Autodesk Inventor part; units mm, degrees
ref_plane "YZ Plane" through (0, 0, 0) normal (1, 0, 0) x (0, 1, 0)
ref_plane "XZ Plane" through (0, 0, 0) normal (0, 1, 0) x (-1, 0, 0)
ref_plane "XY Plane" through (0, 0, 0) normal (0, 0, 1) x (1, 0, 0)
sketch "Sketch1" plane through (0, 0, 0) normal (0, 0, 1) x (1, 0, 0)
  circle A0 centre (0, 0) radius 11.4
  line L0 (-15, 17.5) -> (15, 17.5)
  line L1 (15, 17.5) -> (15, -17.5)
  line L2 (15, -17.5) -> (-15, -17.5)
  line L3 (-15, -17.5) -> (-15, 17.5)
  line L4 (-15, 17.5) -> (15, -17.5) construction
  line L5 (15, 17.5) -> (-15, -17.5) construction
  dimension "d0" = 22.8
  dimension "d1" = 30
  dimension "d2" = 35
extrude "Extrusion1" add sketch "Sketch1" along normal blind 25
sketch "Sketch3" plane through (-15, 17.5, 0) normal (0, 1, 0) x (1, 0, 0)
  line L0 (30, 0) -> (0, 0)
  line L1 (0, 0) -> (30, -25)
  line L2 (45, 40) -> (-15, 40)
  line L3 (-15, 40) -> (-15, -25)
  line L4 (-15, -25) -> (45, -25)
  line L5 (45, -25) -> (45, 40)
  line L6 (0, 0) -> (30, 0)
  line L7 (30, 0) -> (45, 0)
  line L8 (30, -25) -> (0, -25)
  point P0 (15, 0)
  point P1 (15, -12.5)
  dimension "d8" = 60
  dimension "d9" = 65
  dimension "d27" = 0
extrude "Extrusion3" add sketch "Sketch3" along normal blind 6
sketch "Sketch4" plane through (-15, 23.5, 0) normal (0, 1, 0) x (1, 0, 0)
  line L0 (-15, 33) -> (45, 33)
  line L1 (-15, 27) -> (45, 27)
  line L2 (45, 33) -> (45, 27)
  line L3 (-15, 27) -> (-15, 33)
  line L4 (45, 40) -> (-15, 40)
  dimension "d20" = 7
  dimension "d21" = 13
sketch "Sketch5" plane through (0, 0, 25) normal (0, 0, 1) x (1, 0, 0)
  circle A0 centre (0, 0) radius 11.4
  circle A1 centre (0, 0) radius 8.5
  dimension "d24" = 17
extrude "Extrusion5" add sketch "Sketch5" against normal blind 3
chamfer "Chamfer1" distance 5 angle 45 3 edges at (15, 17.5, 12.5) (-15, 17.5, 12.5) (0, 17.5, 0)
extrude "Extrusion6" add sketch "Sketch4" along normal blind 1.5
sketch "Sketch8" plane through (-15, 23.5, 0) normal (0, 1, 0) x (1, 0, 0)
  line L0 (45, 40) -> (-15, 40)
  line L1 (-15, 20) -> (45, 20)
  line L2 (45, 20) -> (45, 14)
  line L3 (45, 14) -> (-15, 14)
  line L4 (-15, 14) -> (-15, 20)
  point P0 (43, 40)
  point P1 (-13, 40)
  point P2 (15, 11.0426)
  dimension "d47" = 6
  dimension "d50" = 20
extrude "Extrusion7" add sketch "Sketch8" along normal blind 20
sketch "Sketch10" plane through (-15, 25, 0) normal (0, 1, 0) x (1, 0, 0)
  line L0 (45, 33) -> (-15, 33)
  line L1 (15, 33) -> (15, 27)
  line L2 (45, 27) -> (-15, 27)
  line L3 (0, 33) -> (0, 27)
  line L4 (30, 33) -> (30, 27)
  point P0 (15, 0)
  point P1 (0, 30)
  point P2 (30, 30)
  dimension "d51" = 15
  dimension "d52" = 15
hole "Hole2" at (-15, 25, -30) at (15, 25, -30) direction (0, -1, 0) diameter 5.5 end through all counterbore diameter 10 counterbore depth 1.5
sketch "Sketch11" plane through (30, 23.5, -20) normal (0, 0, -1) x (-1, 0, 0)
  line L0 (60, 0) -> (60, 20)
  line L1 (60, 10) -> (0, 10)
  line L2 (0, 0) -> (0, 20)
  line L3 (60, 20) -> (0, 20)
  line L4 (30, 20) -> (30, 10)
  point P0 (30, -23.5)
hole "Hole3" at (0, 33.5, -20) direction (0, 0, 1) diameter 5.5 end through all
fillet "Fillet2" radius 2 10 edges at (-30, 20.5, -40) (30, 20.5, -40) (-30, 20.5, 25) (30, 20.5, 25) (30, 43.5, -17) (-30, 43.5, -17) (-15, -17.5, 12.5) (15, -17.5, 12.5) (0, -17.5, 25) (0, -17.5, 0)
properties part number "Estrutura - Suporte Rolamento Z Motor"
Design review of the part built by this model. Coordinates are the model's own, in mm. A direction names the side the tool comes from. Round coordinates to 2 decimals unless told otherwise and drop trailing zeros. Order: outer loops, then holes, each group sorted by start corner. A loop starts at its lowest first (then second) coordinate and runs counter-clockwise, first axis right, second up. Notation, with made-up numbers: M 19,11 L 47,11 A12 cw 47,28 Z; hole C 76,8.25 d7. An arc over 180 degrees is marked long. Answer as CSV lines item,"result". Start each with the question number.
1) Wall thickness on line 1 along X through (y, z) = (18, -30); line 2 along Y through (x, z) = (0, -15); line 3 along Z through (x, y) = (15, 21.9): over which ranges is each line inside the solid? List them lowest first. Write a range as [from, to].
2) Add section D-D (z = -2). Give the boundary of the cut face in (x, y).
3) For pin 1 Ø19.5 at (x, y) = (0, 0) entering from -Z; pin 2 Ø20 at (y, z) = (5, 8.5) entering from +X; pin 3 Ø6 at (x, z) = (-21, -29) entering from -Y, all flat-tipped, find the tip position at first contact; note any pin that passes through.
4) The part is to be moulded in two halves that separate along X. For faces 4 (the face through (-25, 25, -30)), 5 (the face through (15, -1, 12)), 6 (the face through (-9, 7, 11)), say which applies: +X half, -X half, draft (parallel to the pull), parting line (faces both ways), or undercut.
5) Add section C-C (x = -6). Give the boundary of the cut face in (y, z).
6) Add section A-A (y = 0). Give the boundary of the cut face in (x, z), then the cut area to 3 significant figures.
7) Add section B-B (x = 0). Give the number of separate pieces and of enclosed holes in the cut face, then the cut area to 3 significant figures.
8) Tool access review of faces 1 (the face through (0, 25, -30)), 2 (the face through (-4, -8, 22)), 3 (the face through (-7, -11, 0)): name each direction out of +Z, -Z, +X, -X, +Y, -Y from which nothing blocks a thin tool from reaching the whole face with its end or side.
Resolved:
1,line 1,"[-30, -17.75], [-12.25, 12.25], [17.75, 30]"
1,line 2,"[17.5, 30.75], [36.25, 43.5]"
1,line 3,"[-40, -32.75], [-27.25, 25]"
2,outline,"M -30,17.5 L -20,17.5 L -17,14.5 L 17,14.5 L 20,17.5 L 30,17.5 L 30,23.5 L -30,23.5 Z"
3,pin 1,"z = 22"
3,pin 2,"x = 17.5"
3,pin 3,"y = 17.5"
4,face 4,"draft"
4,face 5,"+X half"
4,face 6,"undercut"
5,outline,"M -17.5,2 A2 ccw -15.5,0 L -9.69,0 L -9.69,22 L -6.02,22 L -6.02,25 L -15.5,25 A2 ccw -17.5,23 Z; M 6.02,22 L 9.69,22 L 9.69,0 L 12.5,0 L 17.5,-5 L 17.5,-40 L 23.5,-40 L 23.5,-33 L 25,-33 L 25,-27 L 23.5,-27 L 23.5,-20 L 43.5,-20 L 43.5,-14 L 23.5,-14 L 23.5,25 L 6.02,25 Z"
6,outline,"M -15,0 L -11.4,0 L -11.4,22 L -8.5,22 L -8.5,25 L -15,25 Z; M 8.5,22 L 11.4,22 L 11.4,0 L 15,0 L 15,25 L 8.5,25 Z"
6,area,"197 mm^2"
7,separate pieces,"3"
7,enclosed holes,"0"
7,area,"819 mm^2"
8,face 1,"-Z, +X, -X, +Y"
8,face 2,"-Z"
8,face 3,"-Z, +X, -X, -Y"
